```python
from build123d import *

# Parameters (mm, degrees)
F0_W     = 111
F0_H     = 144.5
F0_R     = 5.25
F0_R_2   = 22.604298
F1_DEPTH = 10
F2_SIZE  = 0.5
F3_R     = 1
F4_SIZE  = 0.5


with BuildPart() as f1:
    # F0 (on Front) → F1 (new body)
    with BuildSketch(Plane.XZ):
        Rectangle(F0_W, F0_H)
        with Locations((-44.25, -58)):
            Circle(F0_R, mode=Mode.SUBTRACT)
        with Locations((0, -13.75)):
            Circle(F0_R_2, mode=Mode.SUBTRACT)
        with Locations((-44.25, 59.5)):
            Circle(F0_R, mode=Mode.SUBTRACT)
        with Locations((44.25, 31)):
            Circle(F0_R, mode=Mode.SUBTRACT)
        with Locations((44.25, 59.5)):
            Circle(F0_R, mode=Mode.SUBTRACT)
    extrude(amount=F1_DEPTH)

    # F2
    f2_edges = [f1.edges().sort_by_distance(p)[0] for p in [
        (0, -10, -72.25),
        (-55.5, -10, 0),
        (0, -10, 72.25),
        (55.5, -10, 0),
        (0, 0, -72.25),
        (55.5, 0, 0),
        (-55.5, 0, 0),
        (0, 0, 72.25),
    ]]
    chamfer(f2_edges, length=F2_SIZE)

    # F3
    f3_edges = [f1.edges().sort_by_distance(p)[0] for p in [
        (55.5, -5, 72.25),
        (55.5, -5, -72.25),
        (-55.5, -5, -72.25),
        (-55.5, -5, 72.25),
    ]]
    fillet(f3_edges, radius=F3_R)

    # F4
    f4_edges = [f1.edges().sort_by_distance(p)[0] for p in [
        (-49.5, 0, 59.5),
        (39, 0, 59.5),
        (39, 0, 31),
        (-49.5, 0, -58),
        (-49.5, -10, 59.5),
        (-49.5, -10, -58),
        (39, -10, 31),
        (39, -10, 59.5),
    ]]
    chamfer(f4_edges, length=F4_SIZE)


solid = f1.part
```
Geometry: final body of the model. Coordinates: model frame, mm. Round coordinates to 2 decimals unless told otherwise and drop trailing zeros. Write each loop counter-clockwise with the first axis right and the second up, starting at its lowest first coordinate (ties: lowest second). Pieces come first, ordered by that corner, then holes. Notation, with made-up numbers: M 72,87 L 111,87 A20 ccw 111,105 Z; hole C 8.25,17.25 d3. An arc over 180 degrees is marked long. Answer in a Markdown table with one row per item. Add a question column.
(1) Cut plane A-A, the plane z = 31. Return the cut outline in (x, y).
(2) Cut plane D-D, the plane x = 14. Return the cut outline in (y, z).
(3) Cut plane C-C, the plane y = -6. Return the cut outline in (x, z), then the cut area to 3 significant figures.
(4) Draft query along X for faces 1 (the face through (-45.388, -4.937, 54.375)), 2 (the face through (-1, -5, -72.25)), 3 (the face through (-55.5, -5, -1)), 4 (the face through (10.431, -4.93, -33.804)). Return one class per face: pulls with the +X half, pulls with the -X half, needs draft (parallel to the pull), parting line crosses it, or undercut.
(5) Ray query, L1, parallel to Z at x = -44.25, y = -4.5; L2, parallel to Z at x = 44.25, y = -4.5; L3, parallel to Z at x = 1, y = -9.5. Return the intervals inside material, ascending.
(6) Cut plane B-B, the plane x = 44.25. Return the cut outline in (y, z), then the cut area to 3 significant figures.
Established:
| question | item | result |
|---|---|---|
| 1 | outline | M -55.5,-9.5 L -55,-10 L 38.5,-10 L 39,-9.5 L 39,-0.5 L 38.5,0 L -55,0 L -55.5,-0.5 Z; M 49.5,-9.5 L 50,-10 L 55,-10 L 55.5,-9.5 L 55.5,-0.5 L 55,0 L 50,0 L 49.5,-0.5 Z |
| 2 | outline | M -10,-71.75 L -9.5,-72.25 L -0.5,-72.25 L 0,-71.75 L 0,-31.5 L -10,-31.5 Z; M -10,4 L 0,4 L 0,71.75 L -0.5,72.25 L -9.5,72.25 L -10,71.75 Z |
| 3 | outline | M -55.5,-71.25 A1 ccw -54.5,-72.25 L 54.5,-72.25 A1 ccw 55.5,-71.25 L 55.5,71.25 A1 ccw 54.5,72.25 L -54.5,72.25 A1 ccw -55.5,71.25 Z; hole C -44.25,-58 d10.5; hole C -44.25,59.5 d10.5; hole C 0,-13.75 d45.21; hole C 44.25,31 d10.5; hole C 44.25,59.5 d10.5 |
| 3 | area | 14,100 mm² |
| 4 | face 1 | undercut |
| 4 | face 2 | needs draft |
| 4 | face 3 | pulls with the -X half |
| 4 | face 4 | undercut |
| 5 | L1 | -72.25 to -63.25, -52.75 to 54.25, 64.75 to 72.25 |
| 5 | L2 | -72.25 to 25.75, 36.25 to 54.25, 64.75 to 72.25 |
| 5 | L3 | -72.25 to -36.33, 8.83 to 72.25 |
| 6 | outline | M -10,-71.75 L -9.5,-72.25 L -0.5,-72.25 L 0,-71.75 L 0,25.25 L -0.5,25.75 L -9.5,25.75 L -10,25.25 Z; M -10,36.75 L -9.5,36.25 L -0.5,36.25 L 0,36.75 L 0,53.75 L -0.5,54.25 L -9.5,54.25 L -10,53.75 Z; M -10,65.25 L -9.5,64.75 L -0.5,64.75 L 0,65.25 L 0,71.75 L -0.5,72.25 L -9.5,72.25 L -10,71.75 Z |
| 6 | area | 1,230 mm² |
